Build history of the part. All positions in model axes, mm. A direction names the side the tool comes from. Round coordinates to 2 decimals unless told otherwise and drop trailing zeros. Write each loop counter-clockwise with the first axis right and the second up, starting at its lowest first coordinate (ties: lowest second). Pieces come first, ordered by that corner, then holes. Notation, with made-up numbers: M -33.5,10 L -8.5,10 A14 cw -8.5,24 Z; hole C 0,40 d7. An arc over 180 degrees is marked long. Write item = value, one per line.
from build123d import *

# Parameters (mm, degrees)
F0_W     = 15
F0_H     = 11
F3_DEPTH = 8.5
F5_R     = 10
F6_DEPTH = 25


# Not quite as in the source:
# - a fillet or chamfer that OpenCascade refuses, or shapes differently, is made with other operations: its cross-section is extruded or revolved along the edge and cut away or added


with BuildPart() as f1:
    # F0 (on Front) → F1 (revolve)
    with BuildSketch(Plane.XZ):
        with Locations((50, 5.5)):
            Rectangle(F0_W, F0_H)
    revolve(axis=Axis((0, 0, 11.3872010261), (0, 0, 1)))

    # F2 (on face) → F3 (cut)
    with BuildSketch(Plane.XY.offset(11)):
        Polygon((-2.0640272124, 46.425), (2.0640272124, 46.425), (4.1280544247, 50), (2.0640272124, 53.575), (-2.0640272124, 53.575), (-4.1280544247, 50), align=None)
        Polygon((-15.8591658515, 43.680976315), (-15.3203466262, 47.7737146618), (-18.5953523929, 50.2867149724), (-22.409177385, 48.7069769362), (-22.9479966103, 44.6142385893), (-19.6729908436, 42.1012382787), align=None)
        Polygon((-31.3679446782, 34.286919955), (-32.4363637825, 38.2743143361), (-36.4237581637, 39.3427334405), (-39.3427334405, 36.4237581637), (-38.2743143361, 32.4363637825), (-34.286919955, 31.3679446782), align=None)
        Polygon((-42.1012382787, 19.6729908436), (-44.6142385893, 22.9479966103), (-48.7069769362, 22.409177385), (-50.2867149724, 18.5953523929), (-47.7737146618, 15.3203466262), (-43.680976315, 15.8591658515), align=None)
        Polygon((-46.425, 2.0640272124), (-50, 4.1280544247), (-53.575, 2.0640272124), (-53.575, -2.0640272124), (-50, -4.1280544247), (-46.425, -2.0640272124), align=None)
        Polygon((-43.680976315, -15.8591658515), (-47.7737146618, -15.3203466262), (-50.2867149724, -18.5953523929), (-48.7069769362, -22.409177385), (-44.6142385893, -22.9479966103), (-42.1012382787, -19.6729908436), align=None)
        Polygon((-34.286919955, -31.3679446782), (-38.2743143361, -32.4363637825), (-39.3427334405, -36.4237581637), (-36.4237581637, -39.3427334405), (-32.4363637825, -38.2743143361), (-31.3679446782, -34.286919955), align=None)
        Polygon((-19.6729908436, -42.1012382787), (-22.9479966103, -44.6142385893), (-22.409177385, -48.7069769362), (-18.5953523929, -50.2867149724), (-15.3203466262, -47.7737146618), (-15.8591658515, -43.680976315), align=None)
        Polygon((-2.0640272124, -46.425), (-4.1280544247, -50), (-2.0640272124, -53.575), (2.0640272124, -53.575), (4.1280544247, -50), (2.0640272124, -46.425), align=None)
        Polygon((15.8591658515, -43.680976315), (15.3203466262, -47.7737146618), (18.5953523929, -50.2867149724), (22.409177385, -48.7069769362), (22.9479966103, -44.6142385893), (19.6729908436, -42.1012382787), align=None)
        Polygon((31.3679446782, -34.286919955), (32.4363637825, -38.2743143361), (36.4237581637, -39.3427334405), (39.3427334405, -36.4237581637), (38.2743143361, -32.4363637825), (34.286919955, -31.3679446782), align=None)
        Polygon((42.1012382787, -19.6729908436), (44.6142385893, -22.9479966103), (48.7069769362, -22.409177385), (50.2867149724, -18.5953523929), (47.7737146618, -15.3203466262), (43.680976315, -15.8591658515), align=None)
        Polygon((46.425, -2.0640272124), (50, -4.1280544247), (53.575, -2.0640272124), (53.575, 2.0640272124), (50, 4.1280544247), (46.425, 2.0640272124), align=None)
        Polygon((43.680976315, 15.8591658515), (47.7737146618, 15.3203466262), (50.2867149724, 18.5953523929), (48.7069769362, 22.409177385), (44.6142385893, 22.9479966103), (42.1012382787, 19.6729908436), align=None)
        Polygon((34.286919955, 31.3679446782), (38.2743143361, 32.4363637825), (39.3427334405, 36.4237581637), (36.4237581637, 39.3427334405), (32.4363637825, 38.2743143361), (31.3679446782, 34.286919955), align=None)
        Polygon((19.6729908436, 42.1012382787), (22.9479966103, 44.6142385893), (22.409177385, 48.7069769362), (18.5953523929, 50.2867149724), (15.3203466262, 47.7737146618), (15.8591658515, 43.680976315), align=None)
    extrude(amount=-F3_DEPTH, mode=Mode.SUBTRACT)

    # F4: fillet of radius 5.5 on 4 edges, made by hand

    # F4_s1 → F4_t2 (revolve, cut)
    with BuildSketch(Plane.XZ):
        with BuildLine():
            ThreePointArc((48, 11), (44.1109127035, 9.3890872965), (42.5, 5.5))
            Line((42.5, 5.5), (42.5, 11))
            Line((42.5, 11), (48, 11))
        make_face()
    revolve(axis=Axis((0, 0, 11), (0, 0, 1)), mode=Mode.SUBTRACT)

    # F4_s3 → F4_t4 (revolve, cut)
    with BuildSketch(Plane.XZ):
        with BuildLine():
            ThreePointArc((52, 11), (55.8890872965, 9.3890872965), (57.5, 5.5))
            Line((57.5, 5.5), (57.5, 11))
            Line((57.5, 11), (52, 11))
        make_face()
    revolve(axis=Axis((0, 0, 11), (0, 0, 1)), mode=Mode.SUBTRACT)

    # F4_s5 → F4_t6 (revolve, cut)
    with BuildSketch(Plane.XZ):
        with BuildLine():
            ThreePointArc((57.5, 5.5), (55.8890872965, 1.6109127035), (52, 0))
            Line((52, 0), (57.5, 0))
            Line((57.5, 0), (57.5, 5.5))
        make_face()
    revolve(axis=Axis((0, 0, 0), (0, 0, 1)), mode=Mode.SUBTRACT)

    # F4_s7 → F4_t8 (revolve, cut)
    with BuildSketch(Plane.XZ):
        with BuildLine():
            ThreePointArc((42.5, 5.5), (44.1109127035, 1.6109127035), (48, 0))
            Line((48, 0), (42.5, 0))
            Line((42.5, 0), (42.5, 5.5))
        make_face()
    revolve(axis=Axis((0, 0, 0), (0, 0, 1)), mode=Mode.SUBTRACT)


with BuildPart() as f6:
    # F5 (on Top) → F6 (new body)
    with BuildSketch(Plane.XY):
        with Locations((0, 50)):
            Circle(F5_R)
    extrude(amount=F6_DEPTH)

    # F7: intersect F1
    add(f1.part, mode=Mode.INTERSECT)


solid = f6.part
1. Mould opens along Y. For faces 3 (the face through (-6, 50, 11)), 4 (the face through (-9.985, 49.456, 5.423)), 5 (the face through (3.11, 51.76, 6.81)) say: pulls with the +Y half, pulls with the -Y half, needs draft (parallel to the pull), parting line crosses it, or undercut.
Responses:
face_3 = needs draft
face_4 = parting line crosses it
face_5 = undercut
2. Flat gauge pins, fed straight in: pin 1 (4 mm diameter, centred on y = 44, z = 2.5, fed in from -X); pin 2 (4.5 mm diameter, centred on x = -0.5, z = 8, fed in from -Y); pin 3 (3.5 mm diameter, centred on x = 0, y = 49.5, fed in from +Z). Where does each tip first touch, or does it go through?
Responses:
pin_1 = -9.17
pin_2 = 42.49
pin_3 = 2.5
3. Tool access for faces 1 (the face through (3.082, 48.187, 6.81)), 2 (the face through (9.97, 49.22, 5.42)): list every direction of +Z, -Z, +X, -X, +Y, -Y with a clear straight run to the whole face (end or side of a thin tool).
Responses:
face_1 = +Z
face_2 = +Z, -Z, +X
4. Band-saw the part on B-B (y = 49.25). List the corners of the cut face in (x, z).
Responses:
outline = M -9.97,0 L 9.97,0 L 9.97,11 L 3.7,11 L 3.7,2.5 L -3.7,2.5 L -3.7,11 L -9.97,11 Z
5. Band-saw the part on A-A (z = 8.5). List the corners of the cut face in (x, y) (3 decimals), plus the area to 3 significant figures.
Responses:
outline = M -7.965,56.047 A10 ccw -6.968,42.827 A43.39 cw 6.968,42.827 A10 ccw 7.965,56.047 A56.61 ccw Z; hole M -4.128,50 L -2.064,46.425 L 2.064,46.425 L 4.128,50 L 2.064,53.575 L -2.064,53.575 Z
area = 200 mm²
6. Probe probe 1 along X at (y, z) = (48, 10); probe 2 along Z at (x, y) = (-3.5, 49); probe 3 along Y at (x, z) = (1.5, 8.75) (3 decimals). List the from-to ranges inside material, lowest first.
Responses:
probe_1 = -9.8 to -2.97, 2.97 to 9.8
probe_2 = 0 to 2.5
probe_3 = 43.537 to 46.425, 53.575 to 56.417
